Autodesk Inventor part; units mm, degrees
ref_plane "YZ Plane" through (0, 0, 0) normal (1, 0, 0) x (0, 1, 0)
ref_plane "XZ Plane" through (0, 0, 0) normal (0, 1, 0) x (-1, 0, 0)
ref_plane "XY Plane" through (0, 0, 0) normal (0, 0, 1) x (1, 0, 0)
sketch "Sketch1" plane through (0, 0, 0) normal (0, 0, 1) x (1, 0, 0)
  line L0 (0, 0) -> (127, 0)
  line L1 (127, 0) -> (127, 76.2)
  line L2 (127, 76.2) -> (0, 76.2)
  line L3 (0, 76.2) -> (0, 0)
  circle A0 centre (63.5, 38.1) radius 14.2875
  circle A1 centre (12.7, 63.5) radius 3.2512
  circle A2 centre (12.7, 38.1) radius 3.2512
  circle A3 centre (12.7, 12.7) radius 3.2512
  circle A4 centre (114.3, 63.5) radius 3.2512
  circle A5 centre (114.3, 38.1) radius 3.2512
  circle A6 centre (114.3, 12.7) radius 3.2512
  dimension "d0" = 127
  dimension "d1" = 76.2
  dimension "d2" = 38.1
  dimension "d3" = 63.5
  dimension "d4" = 28.575
  dimension "d5" = 6.5024
  dimension "d6" = 12.7
  dimension "d7" = 12.7
  dimension "d10" = 25.4
  dimension "d19" = 101.6
extrude "Extrusion2" add sketch "Sketch1" along normal blind 5.08
equation "\"d2\" = 0.5 * d1"
properties part number "Bearing Plate Short"
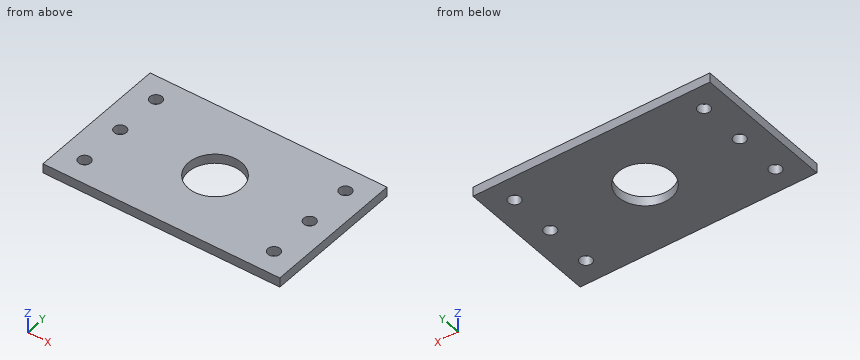
Source: CAD feature listing. Evaluate the final solid. Frame: model axes, mm. Give positions to 0.01 mm unless a question says otherwise; leave off trailing zeros. Order: outer loops, then holes, each group sorted by start corner. A loop starts at its lowest first (then second) coordinate and runs counter-clockwise, first axis right, second up. Notation, with made-up numbers: (-4, -21.75) -> (5, -21.75) arc R20 ccw to (5, 16.25) -> close; hole circle Ø2 at (11.5, 77). An arc over 180 degrees is marked (long way). Use a Markdown table: item, result.
Q1. First-contact query: P1, Ø10, axis at x = 67, y = 41.5, coming from the -Z side. Flat tip, straight axial feed; report the tip coordinate or a pass-through.
A:
| item | result |
|---|---|
| P1 | through |
Q2. Material intervals for line 1 (Y direction, x = 114.3, z = 1.85); line 2 (X direction, y = 65, z = 0.55); line 3 (X direction, y = 61.5, z = 2), sorted ascending. Write a range as [from, to].
A:
| item | result |
|---|---|
| line 1 | [0, 9.45], [15.95, 34.85], [41.35, 60.25], [66.75, 76.2] |
| line 2 | [0, 9.82], [15.58, 111.42], [117.18, 127] |
| line 3 | [0, 10.14], [15.26, 111.74], [116.86, 127] |
Q3. Section A-A (y = 63.5). Return the cut outline in (x, z).
A:
| item | result |
|---|---|
| outline | (0, 0) -> (9.45, 0) -> (9.45, 5.08) -> (0, 5.08) -> close; (15.95, 0) -> (111.05, 0) -> (111.05, 5.08) -> (15.95, 5.08) -> close; (117.55, 0) -> (127, 0) -> (127, 5.08) -> (117.55, 5.08) -> close |
Q4. Section B-B (z = 2.35). Return the cut outline in (x, y) (1 decimal), and give its area (3 significant figures).
A:
| item | result |
|---|---|
| outline | (0, 0) -> (127, 0) -> (127, 76.2) -> (0, 76.2) -> close; hole circle Ø6.5 at (12.7, 12.7); hole circle Ø6.5 at (12.7, 38.1); hole circle Ø6.5 at (12.7, 63.5); hole circle Ø28.6 at (63.5, 38.1); hole circle Ø6.5 at (114.3, 12.7); hole circle Ø6.5 at (114.3, 38.1); hole circle Ø6.5 at (114.3, 63.5) |
| area | 8,840 mm^2 |
Q5. Section C-C (x = 63.5). Return the cut outline in (y, z).
A:
| item | result |
|---|---|
| outline | (0, 0) -> (23.81, 0) -> (23.81, 5.08) -> (0, 5.08) -> close; (52.39, 0) -> (76.2, 0) -> (76.2, 5.08) -> (52.39, 5.08) -> close |
Q6. Section D-D (y = 38.1). Return the cut outline in (x, z).
A:
| item | result |
|---|---|
| outline | (0, 0) -> (9.45, 0) -> (9.45, 5.08) -> (0, 5.08) -> close; (15.95, 0) -> (49.21, 0) -> (49.21, 5.08) -> (15.95, 5.08) -> close; (77.79, 0) -> (111.05, 0) -> (111.05, 5.08) -> (77.79, 5.08) -> close; (117.55, 0) -> (127, 0) -> (127, 5.08) -> (117.55, 5.08) -> close |
